from build123d import *

# Parameters (mm, degrees)
SKETCH_1_R      = 1.5
SKETCH_1_W      = 2
SKETCH_1_H      = 10
EXTRUDE_1_DEPTH = 10


with BuildPart() as part:
    # 草图1 → 凸台-拉伸1 (new body)
    with BuildSketch(Plane(origin=(0, 0, 0), x_dir=(1, 0, 0), z_dir=(0, 1, 0))):
        Polygon((-68, 25), (-47.9, 25), (-11.972426803, 57.430508537), (-47.9, 89.910872233), (-68, 89.910872233), (-70, 89.910872233), (-70, 91.910872233), (-70, 107.910872233), (-70, 109.910872233), (-68, 109.910872233), (-24, 109.910872233), (-24, 114.855181995), (-24, 122.684078109), (-50, 122.684078109), (-50, 137.684078109), (50, 137.684078109), (50, 122.684078109), (24, 122.684078109), (24, 114.855181995), (24, 109.910872233), (68, 109.910872233), (70, 109.910872233), (70, 107.910872233), (70, 91.910872233), (70, 89.910872233), (68, 89.910872233), (48.1, 89.910872233), (12.022357286, 57.385438113), (47.9, 25), (68, 25), (70, 25), (70, 23), (70, -23), (70, -25), (68, -25), (-68, -25), (-70, -25), (-70, -23), (-70, 23), (-70, 25), align=None)
        with Locations((-61.207159892, 12.346732779)):
            Circle(SKETCH_1_R, mode=Mode.SUBTRACT)
        with Locations((-37.207159892, 12.346732779)):
            Circle(SKETCH_1_R, mode=Mode.SUBTRACT)
        with Locations((-37.207159892, -17.653267221)):
            Circle(SKETCH_1_R, mode=Mode.SUBTRACT)
        with Locations((-61.207159892, -17.653267221)):
            Circle(SKETCH_1_R, mode=Mode.SUBTRACT)
        with Locations((61.207159892, -17.653267221)):
            Circle(SKETCH_1_R, mode=Mode.SUBTRACT)
        with Locations((37.207159892, -17.653267221)):
            Circle(SKETCH_1_R, mode=Mode.SUBTRACT)
        with Locations((37.207159892, 12.346732779)):
            Circle(SKETCH_1_R, mode=Mode.SUBTRACT)
        with Locations((61.207159892, 12.346732779)):
            Circle(SKETCH_1_R, mode=Mode.SUBTRACT)
        with Locations((-20.5, 99.910872233)):
            Circle(SKETCH_1_R, mode=Mode.SUBTRACT)
        with Locations((20.5, 99.910872233)):
            Circle(SKETCH_1_R, mode=Mode.SUBTRACT)
        with Locations((-25.210114711, 18.628541516)):
            Circle(SKETCH_1_R, mode=Mode.SUBTRACT)
        with Locations((25.210114711, 18.628541516)):
            Circle(SKETCH_1_R, mode=Mode.SUBTRACT)
        with Locations((-25.210114711, -17.653267221)):
            Circle(SKETCH_1_R, mode=Mode.SUBTRACT)
        with Locations((25.210114711, -17.653267221)):
            Circle(SKETCH_1_R, mode=Mode.SUBTRACT)
        with Locations((6, 130.50199448)):
            Rectangle(SKETCH_1_W, SKETCH_1_H, mode=Mode.SUBTRACT)
        with Locations((-6, 130.50199448)):
            Rectangle(SKETCH_1_W, SKETCH_1_H, mode=Mode.SUBTRACT)
        with Locations((28, 130.50199448)):
            Rectangle(SKETCH_1_W, SKETCH_1_H, mode=Mode.SUBTRACT)
        with Locations((45, 130.50199448)):
            Rectangle(SKETCH_1_W, SKETCH_1_H, mode=Mode.SUBTRACT)
        with Locations((-45, 130.50199448)):
            Rectangle(SKETCH_1_W, SKETCH_1_H, mode=Mode.SUBTRACT)
        with Locations((-28, 130.50199448)):
            Rectangle(SKETCH_1_W, SKETCH_1_H, mode=Mode.SUBTRACT)
        Polygon((-23.789706762, 89.711680759), (23.789706762, 89.711680759), (0, 68.237581075), align=None, mode=Mode.SUBTRACT)
        Polygon((-23.9, 25), (0.033240612, 46.576771159), (23.9, 25), align=None, mode=Mode.SUBTRACT)
    extrude(amount=EXTRUDE_1_DEPTH)


solid = part.part
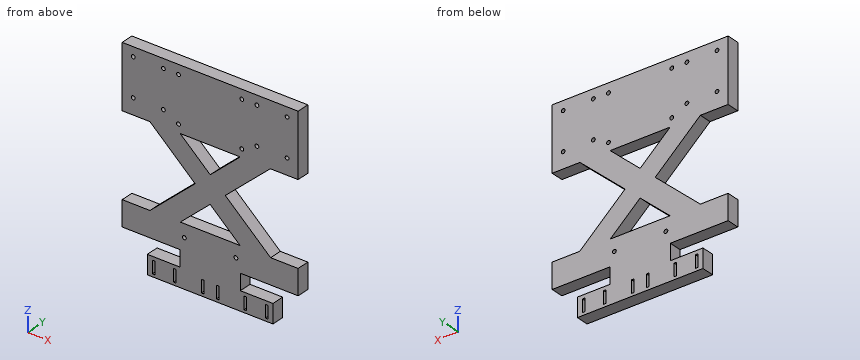
For this review, take the finished solid that the model builds, in its own axes (mm). Round coordinates to 2 decimals unless told otherwise and drop trailing zeros. Loops run counter-clockwise (first coordinate to the right, second up) from the corner with the lowest first, then second, coordinate; pieces in that order, holes last. Notation, with made-up numbers: (50.5, 68) - (60.5, 68) arc R24 cw to (60.5, 91) - close; hole circle Ø9 at (17.5, -27.75). An arc over 180 degrees is marked (long way). Use one line per item in the form item = value.
1) We need section D-D on z = -54. Write out the cut boundary in (x, y), then the cut area to 3 significant figures.
Solutions:
outline = (-15.77, 0) - (15.77, 0) - (15.77, 10) - (-15.77, 10) - close
area = 315 mm2
2) Clearance check with flat-ended pins moving along their axes: P1, Ø2.5, axis at x = -25.21, z = 17.65, coming from the -Y side; P2, Ø5, axis at y = 2.5, z = -115, coming from the +X side; P3, Ø1, axis at y = 7, z = -116.5, coming from the -X side. State where each tip first meets the part, or that it passes through.
Solutions:
P1 = through
P2 = 24
P3 = -24
3) Wall thickness on probe 1 along X at (y, z) = (6, -18.5); probe 2 along Z at (x, y) = (-48.5, 8.25); probe 3 along Z at (x, y) = (-12.5, 4.5): over which ranges is each line inside the solid? List them lowest first.
Solutions:
probe_1 = -70 to -26.7, -23.72 to 23.72, 26.7 to 70
probe_2 = -137.68 to -122.68, -109.91 to -89.91, -25 to 25
probe_3 = -137.68 to -89.71, -79.52 to -57.91, -56.95 to -35.28, -25 to 25
4) We need section B-B on z = -114. Write out the cut boundary in (x, y), then the cut area to 3 significant figures.
Solutions:
outline = (-24, 0) - (24, 0) - (24, 10) - (-24, 10) - close
area = 480 mm2
5) We need section A-A on x = -17. Write out the cut boundary in (y, z).
Solutions:
outline = (0, -137.68) - (10, -137.68) - (10, -89.71) - (0, -89.71) - close; (0, -83.58) - (10, -83.58) - (10, -61.98) - (0, -61.98) - close; (0, -52.89) - (10, -52.89) - (10, -31.22) - (0, -31.22) - close; (0, -25) - (10, -25) - (10, 25) - (0, 25) - close
6) We need section C-C on y = 8.5. State how many separate pieces and enclosed holes the cut face has, then the cut area to 3 significant figures.
Solutions:
separate_pieces = 1
enclosed_holes = 22
area = 14,600 mm2
